```python
from build123d import *

# Parameters (mm, degrees)
F0_W     = 50
F0_H     = 50
F1_DEPTH = 5
F3_DEPTH = 50
F5_DEPTH = 50
F7_DEPTH = 25
F8_R     = 3


with BuildPart() as f1:
    # F0 (on Front) → F1 (new body)
    with BuildSketch(Plane.XZ):
        with Locations((-25, 25)):
            Rectangle(F0_W, F0_H)
    extrude(amount=F1_DEPTH)

    # F2 (on face) → F3 (cut)
    with BuildSketch(Plane.YZ):
        Polygon((0, 45), (0, 50), (-5, 50), align=None)
    extrude(amount=-F3_DEPTH, mode=Mode.SUBTRACT)

    # F4 (on face) → F5 (cut)
    with BuildSketch(Plane(origin=(0, 0, 0), x_dir=(1, 0, 0), z_dir=(0, 0, -1))):
        Polygon((-45, 0), (-50, 5), (-50, 0), align=None)
        Polygon((-5, 0), (0, 0), (0, 5), align=None)
    extrude(amount=-F5_DEPTH, mode=Mode.SUBTRACT)

    # F6 (on face) → F7 (cut)
    with BuildSketch(Plane(origin=(0, 0, 0), x_dir=(-1, 0, 0), z_dir=(0, 1, 0))):
        Polygon((21, 0), (25, 0), (29, 0), (29, 8), (21, 8), align=None)
    extrude(amount=-F7_DEPTH, mode=Mode.SUBTRACT)

    # F8
    f8_edges = [f1.edges().sort_by_distance(p)[0] for p in [
        (-21, -2.5, 8),
        (-29, -2.5, 8),
    ]]
    fillet(f8_edges, radius=F8_R)


solid = f1.part
```
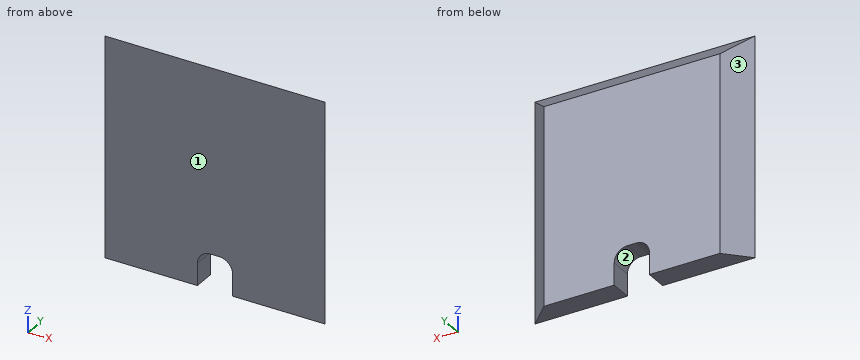
Input: part model. Units: mm. Frame: model coordinates. Face numbers are marked on the shaded views. Coordinates: 2 decimals unless noted, no trailing zeros. Write each loop counter-clockwise with the first axis right and the second up, starting at its lowest first coordinate (ties: lowest second). Pieces come first, ordered by that corner, then holes.
1) Section B-B on x = -10. Output: boundary loops of the cut face in (y, z), and give its area (4 significant figures).
2) Pin query (flat end, axial travel): pin 1 Ø1.5 at (y, z) = (-2.5, 10) entering from +X; pin 2 Ø1 at (x, y) = (-23, -1) entering from -Z; pin 3 Ø1.6 at (x, y) = (-25, -2.5) entering from -Z. Return the tip coordinate at first contact, or that it passes through.
3) Section D-D on z = 10. Output: boundary loops of the cut face in (x, y), and give its area (3 significant figures).
4) Section C-C on y = -3.9. Output: boundary loops of the cut face in (x, z), and give its area (3 significant figures).
5) Mould query, pull axis X, two halves, no side actions, for the marked faces 1, 2 and 3. Classes: pulls with the +X half, pulls with the -X half, needs draft (parallel to the pull), parting line crosses it, or undercut.
6) Section A-A on y = -1.4. Output: boundary loops of the cut face in (x, z), and give its area (3 significant figures).
7) Material intervals for line 1 along X through (y, z) = (-2.9, 5); line 2 along X through (y, z) = (-3.8, 5); line 3 along Z through (x, y) = (-23.5, -3.1), sorted ascending.
Check result:
1. outline: (-5, 0) - (0, 0) - (0, 45) - (-5, 50) - close
1. area: 237.5 mm2
2. pin 1: stops at x = -1.75
2. pin 2: stops at z = 7.6
2. pin 3: stops at z = 8
3. outline: (-50, -5) - (0, -5) - (-5, 0) - (-45, 0) - close
3. area: 225 mm2
4. outline: (-48.9, 0) - (-29, 0) - (-29, 5) arc R3 cw to (-26, 8) - (-24, 8) arc R3 cw to (-21, 5) - (-21, 0) - (-1.1, 0) - (-1.1, 48.9) - (-48.9, 48.9) - close
4. area: 2,280 mm2
5. face 1: needs draft
5. face 2: undercut
5. face 3: pulls with the -X half
6. outline: (-46.4, 0) - (-29, 0) - (-29, 5) arc R3 cw to (-26, 8) - (-24, 8) arc R3 cw to (-21, 5) - (-21, 0) - (-3.6, 0) - (-3.6, 46.4) - (-46.4, 46.4) - close
6. area: 1,930 mm2
7. line 1: x = -47.9 to -29, -21 to -2.1
7. line 2: x = -48.8 to -29, -21 to -1.2
7. line 3: z = 7.96 to 48.1
